CAD build for the part. Positions are in the model's coordinates, mm. Face numbers are marked on the shaded views. A direction names the side the tool comes from. Coordinates: 2 decimals unless noted, no trailing zeros. Order: outer loops, then holes, each group sorted by start corner. A loop starts at its lowest first (then second) coordinate and runs counter-clockwise, first axis right, second up. Notation, with made-up numbers: M 32.5,8.5 L 73.5,8.5 A12 ccw 73.5,19.5 Z; hole C 1.25,50 d2. An arc over 180 degrees is marked long. Write item = value, one per line.
from build123d import *

# Parameters (mm, degrees)
SKETCH017_R      = 1.85
SKETCH017_W      = 1.2
SKETCH017_H      = 4.5
EXTRUDE022_DEPTH = 3
EXTRUDE023_DEPTH = 4.5
EXTRUDE021_DEPTH = 1.5


with BuildPart() as extrude022:
    # Sketch017 (on Face5 of Extrude021) → Extrude022 (new body)
    with BuildSketch(Plane.XZ.offset(-150.4)):
        with Locations((29.2, -30)):
            Circle(SKETCH017_R)
        with Locations((46.5, -30)):
            Circle(SKETCH017_R)
        with Locations((33.95, -30)):
            Rectangle(SKETCH017_W, SKETCH017_H)
        with Locations((41.75, -30)):
            Rectangle(SKETCH017_W, SKETCH017_H)
    extrude(amount=EXTRUDE022_DEPTH)


with BuildPart() as extrude023:
    # Sketch018 (on Face8 of Extrude022) → Extrude023 (new body)
    with BuildSketch(Plane.XY.offset(-27.75)):
        Polygon((33.35, 147.4), (33.35, 149.1), (32.859252, 148.25), align=None)
        Polygon((42.35, 147.4), (42.35, 149.1), (42.840748, 148.25), align=None)
    extrude(amount=-EXTRUDE023_DEPTH)


with BuildPart() as sweep_body:
    # Sweep: sweep along a path in Sketch020
    with BuildLine(Plane.XZ.offset(-150.4)) as sweep_path:
        Line((46.5, -27.25), (29.2, -27.25))
        ThreePointArc((29.200001, -27.25), (26.45, -30), (29.2, -32.75))
        Line((29.2, -32.75), (46.5, -32.75))
        ThreePointArc((46.5, -32.75), (49.25, -29.999999), (46.499999, -27.25))
    # Sketch019 (on Vertex5 of Extrude021) → Sweep (sweep)
    with BuildSketch(Plane(origin=(46.5, 150.4, -27.25), x_dir=(0, 1, 0), z_dir=(1, 0, 0))):
        with BuildLine():
            Line((0.5, 0), (1.5, 0))
            Line((1.5, 0), (1.5, 1))
            ThreePointArc((0.5, 0), (1.207107, 0.292893), (1.5, 1))
        make_face()
    sweep(path=sweep_path.line, is_frenet=True)


with BuildPart() as usb_cover:
    # Sketch016 (on Face14 of Fusion014) → Extrude021 (new body)
    with BuildSketch(Plane(origin=(68, 151.9, 0), x_dir=(-1, 0, 0), z_dir=(0, 1, 0))):
        with BuildLine():
            Line((38.8, -27.25), (21.5, -27.25))
            ThreePointArc((21.5, -27.25), (18.75, -30), (21.5, -32.75))
            Line((38.8, -32.75), (21.5, -32.75))
            ThreePointArc((38.8, -32.75), (41.55, -30), (38.8, -27.25))
        make_face()
    extrude(amount=-EXTRUDE021_DEPTH)

    # Fusion071: union Extrude022, Extrude023, Sweep body
    add(extrude022.part)
    add(extrude023.part)
    add(sweep_body.part)


solid = usb_cover.part
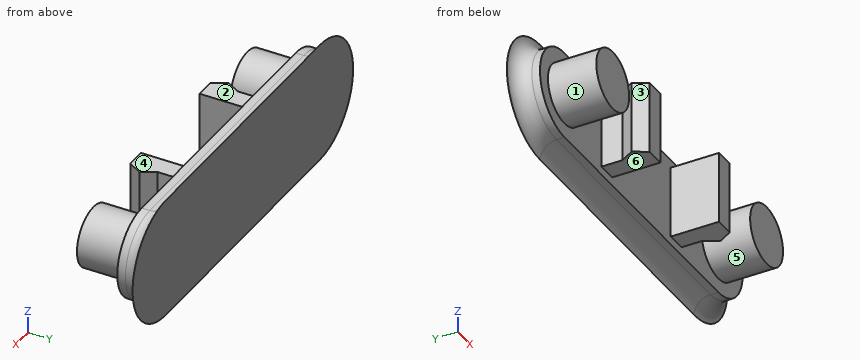
(1) Pull direction X, two halves, no side cores. Call the marked faces 1 and 2: +X half, -X half, draft (parallel to the pull), parting line (faces both ways), or undercut.
Evaluation:
face_1 = undercut
face_2 = draft
(2) Wall check: line 1 (X direction, y = 150.2, z = -30.25); line 2 (X direction, y = 149.6, z = -30.75); line 3 (Z direction, x = 29.25, y = 148.2). Give the ranges that are in metal, low to high. Write a range as from..to.
Evaluation:
line_1 = 27.37..31.03, 33.35..34.55, 41.15..42.35, 44.67..48.33
line_2 = 27.51..30.89, 33.35..34.55, 41.15..42.35, 44.81..48.19
line_3 = -31.85..-28.15
(3) Slice it at A-A, the plane x = 31.75. Write the cut outline in (y, z).
Evaluation:
outline = M 150.4,-32.75 L 150.9,-32.75 A1 cw 151.9,-33.75 L 151.9,-26.25 A1 cw 150.9,-27.25 L 150.4,-27.25 Z
(4) Tool access for the marked faces 3, 4, 5 and 6: list every direction of +Z, -Z, +X, -X, +Y, -Y with a clear straight run to the whole face (end or side of a thin tool).
Evaluation:
face_3 = +Z, -Z, -Y
face_4 = +Z, +X, -X, -Y
face_5 = -Y
face_6 = -Z, +X, -X, -Y
(5) Pin check, flat tips, straight feed: pin 1 Ø2.5 at (y, z) = (148.5, -30) entering from -X; pin 2 Ø2.5 at (y, z) = (148, -29.5) entering from +X; pin 3 Ø0.5 at (x, y) = (34, 149) entering from -Z. Stop position of each tip, or through.
Evaluation:
pin_1 = 27.35
pin_2 = 48.35
pin_3 = -32.25
